Design review of the part built by this model. Coordinates are the model's own, in mm. Face numbers are marked on the shaded views. Round coordinates to 2 decimals unless told otherwise and drop trailing zeros. Loops run counter-clockwise (first coordinate to the right, second up) from the corner with the lowest first, then second, coordinate; pieces in that order, holes last. Notation, with made-up numbers: M 26.25,83 L 85.25,83 A21 ccw 85.25,120 Z; hole C -40,16 d10. An arc over 180 degrees is marked long. One line per item, written item: value. Start each with the question number.
Item 1: We need section B-B (y = -4.25). Write out the cut boundary in (x, z).
Item 2: We need section D-D (x = 1.2). Write out the cut boundary in (y, z).
Item 3: Mouldability with a two-part tool opening along Y and no side actions: class the marked faces 1, 2, 3 and 4 as released by +Y, released by -Y, zero draft, split by the parting line, or undercut.
Item 4: We need section C-C (z = 1.1). Write out the cut boundary in (x, y).
Item 5: We need section A-A (x = 0). Write out the cut boundary in (y, z), then the cut area to 3 significant figures.
Item 6: For line 1 along Y through (x, z) = (0, 1.05); line 2 along Z through (x, y) = (1.7, -1.5); line 3 along Y through (x, z) = (0.8, 1.2), list the stretches that pass through material, from the lowest coordinate up.
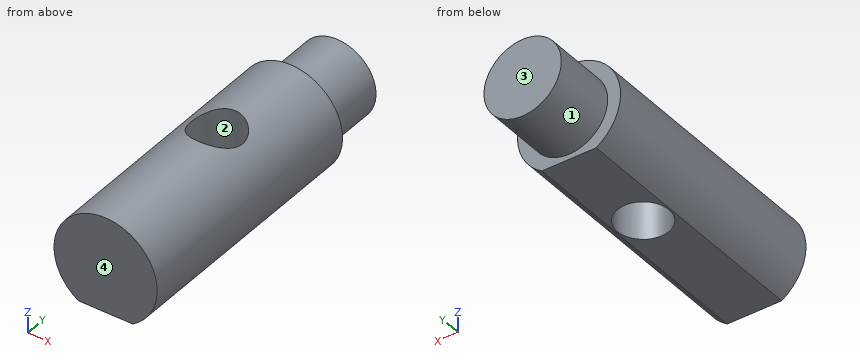
Autodesk Inventor part; units mm, degrees
ref_plane "YZ Plane" through (0, 0, 0) normal (1, 0, 0) x (0, 1, 0)
ref_plane "XZ Plane" through (0, 0, 0) normal (0, 1, 0) x (-1, 0, 0)
ref_plane "XY Plane" through (0, 0, 0) normal (0, 0, 1) x (1, 0, 0)
sketch "スケッチ1" plane through (0, 0, 0) normal (0, 1, 0) x (-1, 0, 0)
  circle A0 centre (0, 0) radius 1.5
  dimension "d0" = 3
extrude "押し出し1" add sketch "スケッチ1" along normal blind 2.5
thread "ねじ1"
sketch "スケッチ2" plane through (0, 0, 0) normal (0, -1, 0) x (1, 0, 0)
  circle A0 centre (0, 0) radius 2
  line L0 (0, -2) -> (0, -1.7)
  line L1 (0, -1.7) -> (-1.0536, -1.7)
  line L2 (0, -1.7) -> (1.0536, -1.7)
  dimension "d5" = 4
  dimension "d6" = 0.3
extrude "押し出し2" add sketch "スケッチ2" along normal blind 10 contours A0 L2 L1
sketch "スケッチ3" plane through (1.0536, 0, -1.7) normal (0, 0, -1) x (-1, 0, 0)
  circle A0 centre (1.0536, -4) radius 1
  line L0 (2.1071, 0) -> (0, 0)
  point P0 (1.0536, 0)
  dimension "d9" = 2
  dimension "d10" = 4
extrude "押し出し3" cut sketch "スケッチ3" against normal blind 10
properties part number "shaftcranp"
A:
1. outline: M -1.05,-1.7 L -0.97,-1.7 L -0.97,1.75 A2 ccw Z; M 0.97,-1.7 L 1.05,-1.7 A2 ccw 0.97,1.75 Z
2. outline: M -10,-1.6 L 0,-1.6 L 0,-0.9 L 2.5,-0.9 L 2.5,0.9 L 0,0.9 L 0,1.6 L -10,1.6 Z
3. face 1: zero draft
3. face 2: undercut
3. face 3: released by +Y
3. face 4: released by -Y
4. outline: M -1.67,-10 L 1.67,-10 L 1.67,0 L 1.02,0 L 1.02,2.5 L -1.02,2.5 L -1.02,0 L -1.67,0 Z; hole C 0,-4 d2
5. outline: M -10,-1.7 L -5,-1.7 L -5,2 L -10,2 Z; M -3,-1.7 L 0,-1.7 L 0,-1.5 L 2.5,-1.5 L 2.5,1.5 L 0,1.5 L 0,2 L -3,2 Z
5. area: 37.1 mm2
6. line 1: -10 to -5, -3 to 2.5
6. line 2: -1.05 to 1.05
6. line 3: -10 to -4.6, -3.4 to 2.5
